For this review, take the finished solid that the model builds, in its own axes (mm). Face numbers are marked on the shaded views. A direction names the side the tool comes from. Give positions to 0.01 mm unless a question says otherwise; leave off trailing zeros. Write each loop counter-clockwise with the first axis right and the second up, starting at its lowest first coordinate (ties: lowest second). Pieces come first, ordered by that corner, then holes.
1) Machinability: for the marked faces 1 and 2, which of the approach directions +Z, -Z, +X, -X, +Y, -Y give a long, thin tool a straight path to every point of the face, cutting with its end or side? Answer none if there is none.
2) Wall thickness on line 1 along Z through (x, y) = (0, -5); line 2 along Z through (x, y) = (-0.75, 3.75); line 3 along Y through (x, z) = (2, 8.75): over which ranges is each line inside the solid? List them lowest first.
3) Draft analysis for pull direction Y (two halves, no side actions). For the marked faces 3, 4 and 5, state which applies: pulls with the +Y half, pulls with the -Y half, needs draft (parallel to the pull), parting line crosses it, or undercut.
4) We need section A-A on x = 0. Give the number of separate pieces and of enclosed holes in the cut face, and give its area (3 significant figures).
5) For P1, Ø5, axis at y = -3, z = 16.5, coming from the +X side; P2, Ø1.2, axis at x = 2.5, z = 4.5, coming from the -Y side; P3, Ø3, axis at x = -3.5, z = 15.5, coming from the +Y side, all flat-tipped, find the tip position at first contact; note any pin that passes through.
6) We need section B-B on z = 3. Give the boundary of the cut face in (x, y).
7) We need section D-D on y = -1.75. Give the boundary of the cut face in (x, z).
from build123d import *

# Parameters (mm, degrees)
F0_R     = 8
F1_DEPTH = 20
F3_DEPTH = 8
F5_D     = 2
F5_DEPTH = 6.001
F7_D     = 2
F8_R     = 2
F9_R     = 1.9999


# Not quite as in the source:
# - a fillet or chamfer is up to 0.001 mm smaller than in the source, because OpenCascade refuses the exact size


with BuildPart() as f1:
    # F0 (on Top) → F1 (new body)
    with BuildSketch(Plane.XY):
        Circle(F0_R)
    extrude(amount=F1_DEPTH)

    # F2 (on face) → F3 (cut)
    with BuildSketch(Plane.XY):
        with BuildLine():
            ThreePointArc((8, 0), (7.9362375701, 1.0080343399), (7.7459666924, 2))
            Line((7.7459666924, 2), (-7.7459666924, 2))
            ThreePointArc((-7.7459666924, 2), (-7.9362375701, 1.0080343399), (-8, 0))
            ThreePointArc((-8, 0), (-7.9362375701, -1.0080343399), (-7.7459666924, -2))
            Line((-7.7459666924, -2), (7.7459666924, -2))
            ThreePointArc((7.7459666924, -2), (7.9362375701, -1.0080343399), (8, 0))
        make_face()
    extrude(amount=F3_DEPTH, mode=Mode.SUBTRACT)

    # F5 (through all, one way)
    with BuildSketch(Plane(origin=(0, -2, 0), x_dir=(-1, 0, 0), z_dir=(0, 1, 0))):
        with Locations((0, 3)):
            Circle(F5_D / 2)
    extrude(amount=-F5_DEPTH, mode=Mode.SUBTRACT)

    # F7 (through all)
    with Locations(Plane.XZ.offset(-2)):
        with Locations((0, 3)):
            Hole(F7_D / 2)

    # F8
    f8_edges = [f1.edges().sort_by_distance(p)[0] for p in [
        (0, 2, 0),
        (0, -2, 0),
    ]]
    fillet(f8_edges, radius=F8_R)

    # F9 (radius 2 in the source; OpenCascade refuses exactly that, so slightly less here)
    f9_edges = [f1.edges().sort_by_distance(p)[0] for p in [
        (0, 2, 8),
        (0, -2, 8),
    ]]
    fillet(f9_edges, radius=F9_R)


solid = f1.part
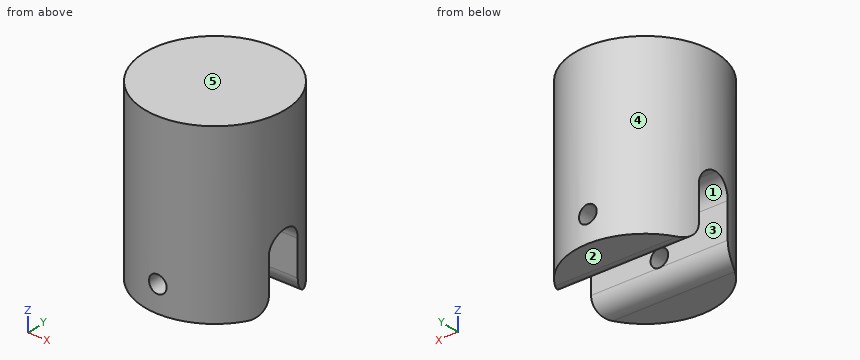
Results list:
1. face 1: -Z, +X, -X
1. face 2: -Z, +X, -X, +Y, -Y
2. line 1: z = 0 to 2, 4 to 20
2. line 2: z = 0.02 to 2.34, 3.66 to 20
2. line 3: y = -7.75 to 7.75
3. face 3: undercut
3. face 4: parting line crosses it
3. face 5: needs draft
4. separate pieces: 3
4. enclosed holes: 0
4. area: 264 mm2
5. P1: stops at x = 7.98
5. P2: stops at y = -7.77
5. P3: stops at y = 7.75
6. outline: (-7.75, -2) arc R8 ccw to (-1, -7.94) - (-1, -2) - close; (-7.75, 2) - (-1, 2) - (-1, 7.94) arc R8 ccw to start; (1, -7.94) arc R8 ccw to (7.75, -2) - (1, -2) - close; (1, 2) - (7.75, 2) arc R8 ccw to (1, 7.94) - close
7. outline: (-7.81, 6.97) - (7.81, 6.97) - (7.81, 20) - (-7.81, 20) - close
